from build123d import *

# Parameters (mm, degrees)
F0_W           = 51
F0_H           = 29
F1_DEPTH       = 5
F3_D           = 4.4
F3_DEPTH       = 6
F3_CBORE_D     = 8.25
F3_CBORE_DEPTH = 4
F3_TIP         = 1.3218933619
F5_D           = 3.3


with BuildPart() as f1:
    # F0 (on Top) → F1 (new body)
    with BuildSketch(Plane.XY):
        Rectangle(F0_W, F0_H)
    extrude(amount=F1_DEPTH)

    # F3
    with Locations(Plane.XY.offset(5)):
        with Locations((-18.5, 9), (-18.5, -9), (11.5, 0)):
            CounterBoreHole(F3_D / 2, F3_CBORE_D / 2, F3_CBORE_DEPTH, depth=F3_DEPTH)
            with Locations((0, 0, -(F3_DEPTH + F3_TIP / 2))):  # 118° drill point
                Cone(0, F3_D / 2, F3_TIP, mode=Mode.SUBTRACT)

    # F5 (through all)
    with Locations(Plane.XY.offset(5)):
        with Locations((-3.5, 9), (-3.5, -9)):
            Hole(F5_D / 2)


solid = f1.part
Geometry check sheet. Reference: the model listing, model coordinates, mm. A direction names the side the tool comes from. Give positions to 0.01 mm unless a question says otherwise; leave off trailing zeros. Order: outer loops, then holes, each group sorted by start corner. A loop starts at its lowest first (then second) coordinate and runs counter-clockwise, first axis right, second up. Notation, with made-up numbers: (8.5, 2.25) - (40.5, 2.25) arc R27 cw to (40.5, 29.25) - close; hole circle Ø8 at (-23.75, -12.75). An arc over 180 degrees is marked (long way). Answer as a JSON object with one key per item and string values.
(1) Cross-section at C-C (x = 11.5). Record the cut outline in (y, z) (3 decimals), then the cut area to 3 significant figures.
Report:
{"outline": "(-14.5, 0) - (-2.2, 0) - (-2.2, 1) - (-4.125, 1) - (-4.125, 5) - (-14.5, 5) - close; (2.2, 0) - (14.5, 0) - (14.5, 5) - (4.125, 5) - (4.125, 1) - (2.2, 1) - close", "area": "108 mm^2"}
(2) Cross-section at B-B (y = 0). Record the cut outline in (x, z) (3 decimals).
Report:
{"outline": "(-25.5, 0) - (9.3, 0) - (9.3, 1) - (7.375, 1) - (7.375, 5) - (-25.5, 5) - close; (13.7, 0) - (25.5, 0) - (25.5, 5) - (15.625, 5) - (15.625, 1) - (13.7, 1) - close"}
(3) Tool access check on faces 4 (the flat face through (0, 0, 0)), 5 (the flat face through (-17, 7, 1)). Record the directions out of +Z, -Z, +X, -X, +Y, -Y that give a thin tool (end or side, any length) a straight path to the whole face; none if there is none.
Report:
{"face 4": "-Z, +X, -X, +Y, -Y", "face 5": "+Z"}
(4) Cross-section at D-D (z = 2.15). Record the cut outline in (x, y) (3 decimals).
Report:
{"outline": "(-25.5, -14.5) - (25.5, -14.5) - (25.5, 14.5) - (-25.5, 14.5) - close; hole circle Ø8.25 at (-18.5, -9); hole circle Ø8.25 at (-18.5, 9); hole circle Ø3.3 at (-3.5, -9); hole circle Ø3.3 at (-3.5, 9); hole circle Ø8.25 at (11.5, 0)"}
(5) Cross-section at A-A (x = -3.5). Record the cut outline in (y, z).
Report:
{"outline": "(-14.5, 0) - (-10.65, 0) - (-10.65, 5) - (-14.5, 5) - close; (-7.35, 0) - (7.35, 0) - (7.35, 5) - (-7.35, 5) - close; (10.65, 0) - (14.5, 0) - (14.5, 5) - (10.65, 5) - close"}
(6) Material ranges on line 1 (Y direction, x = -3.5, z = 3.75); line 2 (Y direction, x = 11.5, z = 2) (3 decimals); line 3 (X direction, y = -9.75, z = 1.8), recorded low to high.
Report:
{"line 1": "-14.5 to -10.65, -7.35 to 7.35, 10.65 to 14.5", "line 2": "-14.5 to -4.125, 4.125 to 14.5", "line 3": "-25.5 to -22.56, -14.44 to -4.97, -2.03 to 25.5"}
(7) Draft check along Y on faces 1 (the cylindrical face through (-21.773, -11.51, 3.028)), 2 (the flat face through (0, 14.5, 2)), 3 (the flat face through (0, -14.5, 2)). Enter one of: released by +Y, released by -Y, zero draft, split by the parting line, or undercut.
Report:
{"face 1": "undercut", "face 2": "released by +Y", "face 3": "released by -Y"}
